from build123d import *

# Parameters (mm, degrees)
SKETCH_1_R          = 13.5
EXTRUDE_1_DEPTH     = 3
SKETCH_2_R          = 1.45
CUT_EXTRUDE_1_DEPTH = 58.750135626
FILLET_1_R          = 5
CUT_EXTRUDE_2_DEPTH = 58.750135626
FILLET_2_R          = 2


with BuildPart() as part:
    # 草图1 → 凸台-拉伸1 (new body)
    with BuildSketch(Plane.XY):
        with BuildLine():
            Line((-49.85055832, 0), (-49.85055832, -15))
            ThreePointArc((-49.85055832, -15), (-15.543694916, -25.465682976), (20.14944168, -29))
            ThreePointArc((20.14944168, -29), (41.64944168, -7.5), (20.14944168, 14))
            ThreePointArc((20.14944168, 14), (-15.543694916, 10.465682976), (-49.85055832, 0))
        make_face()
        with Locations((20.14944168, -7.5)):
            Circle(SKETCH_1_R, mode=Mode.SUBTRACT)
    extrude(amount=EXTRUDE_1_DEPTH)

    # 草图2 → 切除-拉伸1 (cut, through all)
    with BuildSketch(Plane.XY.offset(3)):
        with Locations((-39.85055832, -7.5)):
            Circle(SKETCH_2_R)
        with Locations((-29.85055832, -7.5)):
            Circle(SKETCH_2_R)
        with Locations((-19.85055832, -7.5)):
            Circle(SKETCH_2_R)
    extrude(amount=-CUT_EXTRUDE_1_DEPTH, mode=Mode.SUBTRACT)

    # 圆角1
    fillet_1_edges = [part.edges().sort_by_distance(p)[0] for p in [
        (-49.85055832, -15, 1.5),
        (-49.85055832, 0, 1.5),
    ]]
    fillet(fillet_1_edges, radius=FILLET_1_R)

    # 草图3 → 切除-拉伸2 (cut, through all)
    with BuildSketch(Plane.XY.offset(3)):
        with BuildLine():
            Line((-32.310066515, 0), (0, 0))
            ThreePointArc((0, 0), (1.911289465, 3.885069336), (4.562236757, 7.308411215))
            ThreePointArc((4.562236757, 7.308411215), (-14.069588262, 4.641414469), (-32.310066515, 0))
        make_face()
        with BuildLine():
            Line((-32.310066515, -15), (0, -15))
            ThreePointArc((0, -15), (1.911289465, -18.885069336), (4.562236757, -22.308411215))
            ThreePointArc((4.562236757, -22.308411215), (-14.069588262, -19.641414469), (-32.310066515, -15))
        make_face()
    extrude(amount=-CUT_EXTRUDE_2_DEPTH, mode=Mode.SUBTRACT)

    # 圆角2
    fillet_2_edges = [part.edges().sort_by_distance(p)[0] for p in [
        (0, -15, 1.5),
        (4.562236757, -22.308411215, 1.5),
        (-32.310066515, -15, 1.5),
        (4.562236757, 7.308411215, 1.5),
        (0, 0, 1.5),
        (-32.310066515, 0, 1.5),
    ]]
    fillet(fillet_2_edges, radius=FILLET_2_R)


solid = part.part
Work out the finished part from the listing and answer in its coordinate system (mm). A direction names the side the tool comes from. Round coordinates to 2 decimals unless told otherwise and drop trailing zeros. Write each loop counter-clockwise with the first axis right and the second up, starting at its lowest first coordinate (ties: lowest second). Pieces come first, ordered by that corner, then holes. Notation, with made-up numbers: (-23.75, 52.25) - (17.25, 52.25) arc R26 ccw to (17.25, 71.25) - close; hole circle Ø4 at (18, -21.75). An arc over 180 degrees is marked (long way). Answer in a Markdown table with one row per item. Add a question column.
1. A cutting plane is placed at C-C, the plane y = -14. Determine the outline of the cut face in (x, z).
2. For faces 4 (the cylindrical face through (-14.339, -25.702, 1.479)), 5 (the cylindrical face through (1.116, 2.499, 1.521)), determine the directions among +Z, -Z, +X, -X, +Y, -Y from which every point of the face is accessible in a straight line to the end or side of a thin tool.
3. A cutting plane is placed at A-A, the plane y = -7.5. Determine the outline of the cut face in (x, z), and give its area (3 significant figures).
4. Given pin 1 (1 mm diameter, centred on y = 2, z = 1.5, fed in from +X); pin 2 (4 mm diameter, centred on x = 6.5, y = -19.5, fed in from -Z), each flat-ended and moving along its own axis, determine where each tip first touches the part or whether it passes through.
5. A cutting plane is placed at D-D, the plane z = 1.45. Count the separate pieces of the cut face and the enclosed holes in it, and give its area (3 significant figures).
6. Find the intervals of material crossed by line 1 along Y through (x, z) = (-10.5, 0.7); line 2 along Y through (x, z) = (-3.5, 1.7); line 3 along Y through (x, z) = (24, 0.95), in increasing order. Write a range as from..to.
7. The mould has two halves that part along X. Classify faces 1 (the flat face through (-5, -7, 3)), 2 (the cylindrical face through (-49.01, -14.41, 1.52)), 3 (the cylindrical face through (-0.267, 0.315, 1.479)): +X half, -X half, draft (parallel to the pull), parting line (faces both ways), or undercut.
8. A cutting plane is placed at B-B, the plane x = 27. Determine the outline of the cut face in (y, z), and give its area (3 significant figures).
Worked out:
| question | item | result |
|---|---|---|
| 1 | outline | (-49.25, 0) - (8.32, 0) - (8.32, 3) - (-49.25, 3) - close; (31.98, 0) - (40.64, 0) - (40.64, 3) - (31.98, 3) - close |
| 2 | face 4 | +Z, -Z, -X, -Y |
| 2 | face 5 | +Z, -Z |
| 3 | outline | (-49.85, 0) - (-41.3, 0) - (-41.3, 3) - (-49.85, 3) - close; (-38.4, 0) - (-31.3, 0) - (-31.3, 3) - (-38.4, 3) - close; (-28.4, 0) - (-21.3, 0) - (-21.3, 3) - (-28.4, 3) - close; (-18.4, 0) - (6.65, 0) - (6.65, 3) - (-18.4, 3) - close; (33.65, 0) - (41.65, 0) - (41.65, 3) - (33.65, 3) - close |
| 3 | area | 167 mm^2 |
| 4 | pin 1 | x = 39.68 |
| 4 | pin 2 | z = 0 |
| 5 | separate pieces | 1 |
| 5 | enclosed holes | 6 |
| 5 | area | 2,280 mm^2 |
| 6 | line 1 | -26.4..-20.31, -15..0, 5.31..11.4 |
| 6 | line 2 | -27.46..-21.4, -15..0, 6.4..12.46 |
| 6 | line 3 | -28.65..-20.44, 5.44..13.65 |
| 7 | face 1 | draft |
| 7 | face 2 | -X half |
| 7 | face 3 | undercut |
| 8 | outline | (-27.88, 0) - (-19.13, 0) - (-19.13, 3) - (-27.88, 3) - close; (4.13, 0) - (12.88, 0) - (12.88, 3) - (4.13, 3) - close |
| 8 | area | 52.5 mm^2 |
